Check sheet for the modelled part. Datum: model origin and axes. Units: mm. Give positions to 0.01 mm unless a question says otherwise; leave off trailing zeros. Write each loop counter-clockwise with the first axis right and the second up, starting at its lowest first coordinate (ties: lowest second). Pieces come first, ordered by that corner, then holes. Notation, with made-up numbers: M 31,70.5 L 64,70.5 A13 cw 64,78.5 Z; hole C 74.5,85 d4. An arc over 180 degrees is marked long. Write item = value, one per line. Start each with the question number.
1) Draft check along Y on faces 1 (the face through (18.318, -23.234, -2.854)), 2 (the face through (-41.07, -51, -2.54)), 3 (the face through (-42.5, -1, -2)). Enter one of: pulls with the +Y half, pulls with the -Y half, needs draft (parallel to the pull), parting line crosses it, or undercut.
2) Sectioned sample at C-C, the plane y = 0. Record the cut outline in (x, z).
3) Scan lines: L1, parallel to Y at x = -30, z = -0.45; L2, parallel to Y at x = -20, z = -3.55; L3, parallel to X at y = 20, z = -3.7. Record each from-to range of solid material in increasing order.
4) Gauge pin test, flat ends, axial feed: pin 1 (11 mm diameter, centred on x = 20, y = 20, fed in from -Z); pin 2 (9 mm diameter, centred on x = -20, y = -20, fed in from +Z); pin 3 (11 mm diameter, centred on x = -20, y = 20, fed in from +Z); pin 4 (14.5 mm diameter, centred on x = 30, y = 40, fed in from -Z). Record the tip position at first contact, or that the pin passes through.
5) Sectioned sample at D-D, the plane x = 30. Record the cut outline in (y, z), then the cut area to 3 significant figures.
6) Sectioned sample at B-B, the plane y = -40. Record the cut outline in (x, z).
7) Sectioned sample at A-A, the plane x = 0. Record the cut outline in (y, z), then the cut area to 3 significant figures.
from build123d import *

# Parameters (mm, degrees)
F0_W           = 85
F0_H           = 105
F1_DEPTH       = 5
F2_R           = 5.1
F2_R_2         = 4.5
F3_DEPTH       = 5.001
F5_D           = 7
F5_CSINK_D     = 13
F5_CSINK_ANGLE = 90
F6_R           = 5
F7_SIZE        = 4.1


with BuildPart() as f1:
    # F0 (on Top) → F1 (new body)
    with BuildSketch(Plane.XY):
        Rectangle(F0_W, F0_H)
    extrude(amount=-F1_DEPTH)

    # F2 (on face) → F3 (cut, through all)
    with BuildSketch(Plane.XY):
        Circle(F2_R)
        with Locations((30, 40)):
            Circle(F2_R_2)
        with Locations((-30, 40)):
            Circle(F2_R_2)
        with Locations((-30, -40)):
            Circle(F2_R_2)
        with Locations((30, -40)):
            Circle(F2_R_2)
    extrude(amount=-F3_DEPTH, mode=Mode.SUBTRACT)

    # F5 (through all)
    with Locations(Plane.XY):
        with Locations((-20, 20), (20, 20), (20, -20), (-20, -20)):
            CounterSinkHole(F5_D / 2, F5_CSINK_D / 2, counter_sink_angle=F5_CSINK_ANGLE)

    # F6
    f6_edges = [f1.edges().sort_by_distance(p)[0] for p in [
        (-42.5, -52.5, -2.5),
        (42.5, -52.5, -2.5),
        (42.5, 52.5, -2.5),
        (-42.5, 52.5, -2.5),
    ]]
    fillet(f6_edges, radius=F6_R)

    # F7
    f7_edges = [f1.edges().sort_by_distance(p)[0] for p in [
        (25.5, 40, -5),
        (-34.5, 40, -5),
        (-34.5, -40, -5),
        (25.5, -40, -5),
    ]]
    chamfer(f7_edges, length=F7_SIZE)


solid = f1.part
Data:
q1.face_1 = undercut
q1.face_2 = pulls with the -Y half
q1.face_3 = needs draft
q2.outline = M -42.5,-5 L -5.1,-5 L -5.1,0 L -42.5,0 Z; M 5.1,-5 L 42.5,-5 L 42.5,0 L 5.1,0 Z
q3.L1 = -52.5 to -44.5, -35.5 to 35.5, 44.5 to 52.5
q3.L2 = -52.5 to -23.5, -16.5 to 16.5, 23.5 to 52.5
q3.L3 = -42.5 to -23.5, -16.5 to 16.5, 23.5 to 42.5
q4.pin_1 = -5
q4.pin_2 = -2
q4.pin_3 = -1
q4.pin_4 = -3.65
q5.outline = M -52.5,-5 L -48.6,-5 L -44.5,-0.9 L -44.5,0 L -52.5,0 Z; M -35.5,-0.9 L -31.4,-5 L 31.4,-5 L 35.5,-0.9 L 35.5,0 L -35.5,0 Z; M 44.5,-0.9 L 48.6,-5 L 52.5,-5 L 52.5,0 L 44.5,0 Z
q5.area = 401 mm2
q6.outline = M -42.5,-5 L -38.6,-5 L -34.5,-0.9 L -34.5,0 L -42.5,0 Z; M -25.5,-0.9 L -21.4,-5 L 21.4,-5 L 25.5,-0.9 L 25.5,0 L -25.5,0 Z; M 34.5,-0.9 L 38.6,-5 L 42.5,-5 L 42.5,0 L 34.5,0 Z
q7.outline = M -52.5,-5 L -5.1,-5 L -5.1,0 L -52.5,0 Z; M 5.1,-5 L 52.5,-5 L 52.5,0 L 5.1,0 Z
q7.area = 474 mm2
